Verification items for the finished model (mm, model axes). A direction names the side the tool comes from. Round coordinates to 2 decimals unless told otherwise and drop trailing zeros. Order: outer loops, then holes, each group sorted by start corner. A loop starts at its lowest first (then second) coordinate and runs counter-clockwise, first axis right, second up. Notation, with made-up numbers: M 5.25,49.25 L 24.25,49.25 A21 ccw 24.25,78.25 Z; hole C -28.5,-1 d10. An arc over 180 degrees is marked long. Answer as a JSON object with one key per item and string values. Group by question number.
```python
from build123d import *

# Parameters (mm, degrees)
SKETCH1_W           = 106
SKETCH1_H           = 6
SKETCH1_H_2         = 9.4
SKETCH1_H_3         = 8.5
SKETCH1_H_4         = 4.8
BOSS_EXTRUDE4_DEPTH = 4
SKETCH5_W           = 106
SKETCH5_H           = 6
BOSS_EXTRUDE5_DEPTH = 7.6
SKETCH4_W           = 106
SKETCH4_H           = 6
BOSS_EXTRUDE6_DEPTH = 7.6
SKETCH6_R           = 1.75
CUT_EXTRUDE1_DEPTH  = 20
CUT_EXTRUDE3_DEPTH  = 3.5
BOSS_EXTRUDE8_DEPTH = 3
BOSS_EXTRUDE9_DEPTH = 3


with BuildPart() as part:
    # Sketch1 → Boss-Extrude4 (new body)
    with BuildSketch(Plane(origin=(0, 0, 0), x_dir=(1, 0, 0), z_dir=(0, 1, 0))):
        with Locations((53, 20.9)):
            Rectangle(SKETCH1_W, SKETCH1_H)
        with Locations((53, 13.2)):
            Rectangle(SKETCH1_W, SKETCH1_H_2)
        with Locations((53, 4.25)):
            Rectangle(SKETCH1_W, SKETCH1_H_3)
        with Locations((53, -2.4)):
            Rectangle(SKETCH1_W, SKETCH1_H_4)
        with Locations((53, -9.05)):
            Rectangle(SKETCH1_W, SKETCH1_H_3)
        with Locations((53, -18)):
            Rectangle(SKETCH1_W, SKETCH1_H_2)
        with Locations((53, -25.7)):
            Rectangle(SKETCH1_W, SKETCH1_H)
    extrude(amount=BOSS_EXTRUDE4_DEPTH)

    # Sketch5 → Boss-Extrude5 (add)
    with BuildSketch(Plane(origin=(0, 4, 0), x_dir=(1, 0, 0), z_dir=(0, 1, 0))):
        with Locations((53, 20.9)):
            Rectangle(SKETCH5_W, SKETCH5_H)
        with Locations((53, -25.7)):
            Rectangle(SKETCH5_W, SKETCH5_H)
    extrude(amount=BOSS_EXTRUDE5_DEPTH)

    # Sketch4 → Boss-Extrude6 (add)
    with BuildSketch(Plane(origin=(0, 4, 0), x_dir=(1, 0, 0), z_dir=(0, 1, 0))):
        with Locations((53, 20.9)):
            Rectangle(SKETCH4_W, SKETCH4_H)
        with Locations((53, -25.7)):
            Rectangle(SKETCH4_W, SKETCH4_H)
    extrude(amount=BOSS_EXTRUDE6_DEPTH)

    # Sketch6 → Cut-Extrude1 (cut)
    with BuildSketch(Plane(origin=(0, 11.6, 0), x_dir=(1, 0, 0), z_dir=(0, 1, 0))):
        with Locations((92, 20.9)):
            Circle(SKETCH6_R)
        with Locations((92, -25.7)):
            Circle(SKETCH6_R)
        with Locations((14, 20.9)):
            Circle(SKETCH6_R)
        with Locations((14, -25.7)):
            Circle(SKETCH6_R)
    extrude(amount=-CUT_EXTRUDE1_DEPTH, mode=Mode.SUBTRACT)

    # Sketch7 → Cut-Extrude3 (cut)
    with BuildSketch(Plane.XZ):
        Polygon((17.464101615, 25.7), (15.732050808, 28.7), (12.267949192, 28.7), (10.535898385, 25.7), (12.267949192, 22.7), (15.732050808, 22.7), align=None)
        Polygon((95.464101615, 25.7), (93.732050808, 28.7), (90.267949192, 28.7), (88.535898385, 25.7), (90.267949192, 22.7), (93.732050808, 22.7), align=None)
        Polygon((17.464101615, -20.9), (15.732050808, -17.9), (12.267949192, -17.9), (10.535898385, -20.9), (12.267949192, -23.9), (15.732050808, -23.9), align=None)
        Polygon((95.464101615, -20.9), (93.732050808, -17.9), (90.267949192, -17.9), (88.535898385, -20.9), (90.267949192, -23.9), (93.732050808, -23.9), align=None)
    extrude(amount=-CUT_EXTRUDE3_DEPTH, mode=Mode.SUBTRACT)

    # Sketch8 → Boss-Extrude8 (add)
    with BuildSketch(Plane.XY.offset(28.7)):
        Polygon((38, 11.6), (33, 16.6), (63, 16.6), (68, 11.6), align=None)
    extrude(amount=-BOSS_EXTRUDE8_DEPTH)

    # Sketch9 → Boss-Extrude9 (add)
    with BuildSketch(Plane(origin=(0, 0, -23.9), x_dir=(-1, 0, 0), z_dir=(0, 0, -1))):
        Polygon((-68, 11.6), (-63, 16.6), (-33, 16.6), (-38, 11.6), align=None)
    extrude(amount=-BOSS_EXTRUDE9_DEPTH)


solid = part.part
```
Q1. Thickness scan on line 1 (X direction, y = 6.75, z = -20.9); line 2 (Z direction, x = 14, y = 7); line 3 (Z direction, x = 47, y = 13). Record the ranges inside material, lowest first. Write a range as from..to.
Q2. Cross-section at D-D, the plane x = 58. Record the cut outline in (y, z).
Q3. Cross-section at B-B, the plane x = 14. Record the cut outline in (y, z), then the cut area to 3 significant figures.
Q4. Cross-section at C-C, the plane y = 13.5. Record the cut outline in (x, z), then the cut area to 3 significant figures.
Q5. Tool access check on faces 1 (the face through (94.6, 1.7, -22.4)), 2 (the face through (91.772, 7.607, 23.965)), 3 (the face through (14, 2, -17.9)), 4 (the face through (50, 14, -20.9)). Record the directions out of +Z, -Z, +X, -X, +Y, -Y that give a thin tool (end or side, any length) a straight path to the whole face; none if there is none.
Q6. Release check for a two-part mould opening along X. For faces 5 (the face through (94.6, 1.7, 24.2)), 6 (the face through (52, 8, -17.9)) record: released by +X, released by -X, zero draft, split by the parting line, or undercut.
Q7. Cross-section at A-A, the plane y = 7. Record the cut outline in (x, z).
Q8. Gauge pin test, flat ends, axial feed: pin 1 Ø3 at (x, z) = (61.5, 21) entering from -Y; pin 2 Ø1 at (x, y) = (92, 2) entering from -Z; pin 3 Ø5 at (x, z) = (77.5, 25.5) entering from +Y; pin 4 Ø4.5 at (x, z) = (14, 25.7) entering from -Y. Record the tip position at first contact, or that the pin passes through.
Conclusion:
{
 "1": {"line 1": "0..12.25, 15.75..90.25, 93.75..106", "line 2": "-23.9..-22.65, -19.15..-17.9, 22.7..23.95, 27.45..28.7", "line 3": "-23.9..-20.9, 25.7..28.7"},
 "2": {"outline": "M 0,-23.9 L 16.6,-23.9 L 16.6,-20.9 L 11.6,-20.9 L 11.6,-17.9 L 4,-17.9 L 4,22.7 L 11.6,22.7 L 11.6,25.7 L 16.6,25.7 L 16.6,28.7 L 0,28.7 Z"},
 "3": {"outline": "M 0,-17.9 L 3.5,-17.9 L 3.5,-19.15 L 11.6,-19.15 L 11.6,-17.9 L 4,-17.9 L 4,22.7 L 11.6,22.7 L 11.6,23.95 L 3.5,23.95 L 3.5,22.7 L 0,22.7 Z; M 3.5,-23.9 L 11.6,-23.9 L 11.6,-22.65 L 3.5,-22.65 Z; M 3.5,27.45 L 11.6,27.45 L 11.6,28.7 L 3.5,28.7 Z", "area": "203 mm2"},
 "4": {"outline": "M 36.1,-23.9 L 66.1,-23.9 L 66.1,-20.9 L 36.1,-20.9 Z; M 36.1,25.7 L 66.1,25.7 L 66.1,28.7 L 36.1,28.7 Z", "area": "180 mm2"},
 "5": {"face 1": "-Y", "face 2": "+Y, -Y", "face 3": "-Z, -Y", "face 4": "+X, -X, +Y"},
 "6": {"face 5": "undercut", "face 6": "zero draft"},
 "7": {"outline": "M 0,-23.9 L 106,-23.9 L 106,-17.9 L 0,-17.9 Z; M 0,22.7 L 106,22.7 L 106,28.7 L 0,28.7 Z; hole C 14,-20.9 d3.5; hole C 14,25.7 d3.5; hole C 92,-20.9 d3.5; hole C 92,25.7 d3.5"},
 "8": {"pin 1": "y = 0", "pin 2": "z = -17.9", "pin 3": "y = 11.6", "pin 4": "y = 3.5"}
}
